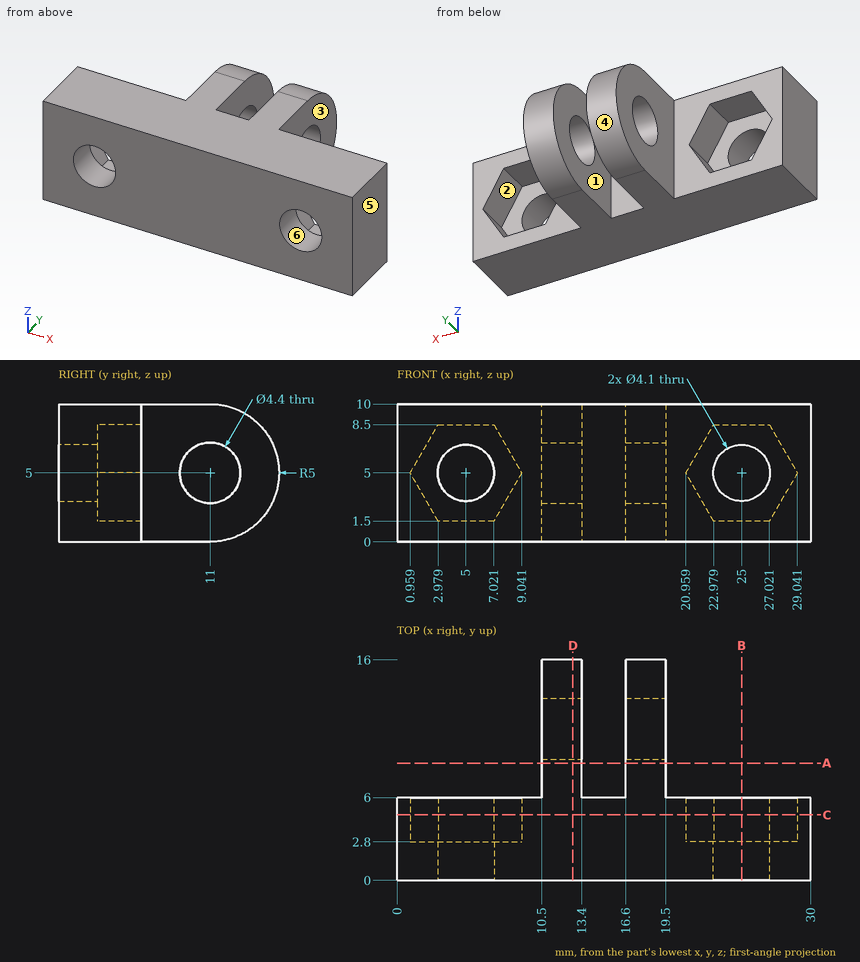
Part print with two shaded views. Sizes in mm from the minimum x, y, z corner. A direction names the side the tool comes from. Coordinates: 2 decimals unless noted, no trailing zeros. Write each loop counter-clockwise with the first axis right and the second up, starting at its lowest first coordinate (ties: lowest second). Pieces come first, ordered by that corner, then holes. Notation, with made-up numbers: (63.25, 9.5) - (91.25, 9.5) arc R20 ccw to (91.25, 41.5) - close; hole circle Ø9 at (-35, -0.5). An arc over 180 degrees is marked (long way). One line per item, written item: value. Start each with the question number.
1. Mould opens along Z. For the marked faces 4, 5 and 6 say: released by +Z, released by -Z, zero draft, split by the parting line, or undercut.
2. Slice it at A-A (y = 8.5). Write the cut outline in (x, z).
3. Tool access for the marked faces 1, 2 and 3: list every direction of +Z, -Z, +X, -X, +Y, -Y with a clear straight run to the whole face (end or side of a thin tool).
4. Probe line 1 (X direction, y = 0.95, z = 5); line 2 (Z direction, x = 18.1, y = 11); line 3 (X direction, y = 6.5, z = 1.5). List the from-to ranges inside material, lowest first. Write a range as from..to.
5. Slice it at D-D (x = 12.75). Write the cut outline in (y, z), plus the area to 3 significant figures.
6. Slice it at B-B (x = 25). Write the cut outline in (y, z).
7. Flat gauge pins, fed straight in: pin 1 (3.5 mm diameter, centred on x = 25.5, z = 6.5, fed in from +Y); pin 2 (3.5 mm diameter, centred on x = 14.5, z = 2.5, fed in from +Y); pin 3 (3 mm diameter, centred on y = 13.5, z = 8.5, fed in from +X). Where does each tip first touch, or does it go through?
8. Slice it at C-C (y = 4.75). Write the cut outline in (x, z), plus the area to 3 significant figures.
Answers below:
1. face 4: split by the parting line
1. face 5: zero draft
1. face 6: undercut
2. outline: (10.5, 0) - (13.4, 0) - (13.4, 10) - (10.5, 10) - close; (16.6, 0) - (19.5, 0) - (19.5, 10) - (16.6, 10) - close
3. face 1: +Z, -Z, +Y
3. face 2: +Y
3. face 3: +Z, -Z, +X, +Y
4. line 1: x = 0..2.95, 7.05..22.95, 27.05..30
4. line 2: z = 0..2.8, 7.2..10
4. line 3: x = 10.5..13.4, 16.6..19.5
5. outline: (0, 0) - (11, 0) arc R5 ccw to (11, 10) - (0, 10) - close; hole circle Ø4.4 at (11, 5)
5. area: 134 mm^2
6. outline: (0, 0) - (6, 0) - (6, 1.5) - (2.8, 1.5) - (2.8, 2.95) - (0, 2.95) - close; (0, 7.05) - (2.8, 7.05) - (2.8, 8.5) - (6, 8.5) - (6, 10) - (0, 10) - close
7. pin 1: stops at y = 2.8
7. pin 2: stops at y = 15.87
7. pin 3: stops at x = 19.5
8. outline: (0, 0) - (30, 0) - (30, 10) - (0, 10) - close; hole (0.96, 5) - (2.98, 1.5) - (7.02, 1.5) - (9.04, 5) - (7.02, 8.5) - (2.98, 8.5) - close; hole (20.96, 5) - (22.98, 1.5) - (27.02, 1.5) - (29.04, 5) - (27.02, 8.5) - (22.98, 8.5) - close
8. area: 215 mm^2
